Input: part model. Units: mm. Frame: model coordinates. A direction names the side the tool comes from. Coordinates: 2 decimals unless noted, no trailing zeros. Write each loop counter-clockwise with the first axis right and the second up, starting at its lowest first coordinate (ties: lowest second). Pieces come first, ordered by that corner, then holes. Notation, with made-up numbers: (6, 0) - (51, 0) arc R23 cw to (51, 19) - close; hole circle Ø9 at (78.5, 29). An arc over 180 degrees is marked (long way). Use CSV: the item, a comma, the result in double quotes.
Autodesk Fusion 360 part; units mm, degrees
sketch "Sketch1" plane through (0, 0, 0) normal (0, 0, 1) x (1, 0, 0)
  line L0 (-50.8, 50.8) -> (50.8, 50.8)
  line L1 (50.8, 50.8) -> (50.8, -50.8)
  line L2 (50.8, -50.8) -> (-50.8, -50.8)
  line L3 (-50.8, -50.8) -> (-50.8, 50.8)
  line L4 (-50.8, 50.8) -> (50.8, -50.8) construction
  line L5 (50.8, 50.8) -> (-50.8, -50.8) construction
  circle A0 centre (0, 0) radius 27.43
  line L6 (0, 0) -> (-40.48, 0) construction
  line L7 (-40.48, 0) -> (-40.48, -40.48) construction
  line L8 (-40.48, -40.48) -> (0, -40.48) construction
  line L9 (0, -40.48) -> (0, 0) construction
  circle A1 centre (-40.48, -40.48) radius 1.985
  circle A2 centre (-40.48, 40.48) radius 1.985
  circle A3 centre (40.48, 40.48) radius 1.985
  circle A4 centre (40.48, -40.48) radius 1.985
  circle A5 centre (0, 0) radius 45
  dimension "d1" = 101.6
  dimension "d2" = 101.6
  dimension "d3" = 54.86
  dimension "d4" = 40.48
  dimension "d5" = 40.48
  dimension "d6" = 3.97
extrude "Extrude1" add sketch "Sketch1" against normal blind 0.74 contours L0 L1 L2 L3 | A5
extrude "Extrude2" add sketch "Sketch1" along normal blind 6.65 contours A5
sketch "Sketch2" plane through (0, 0, 6.65) normal (0, 0, 1) x (-1, 0, 0)
  circle A0 centre (0, 0) radius 27.43
  circle A1 centre (0, 0) radius 45
  circle A2 centre (0, 0) radius 45
  circle A3 centre (-40.48, 40.48) radius 1.985
  circle A4 centre (40.48, 40.48) radius 1.985
  circle A5 centre (40.48, -40.48) radius 1.985
  circle A6 centre (-40.48, -40.48) radius 1.985
  line L0 (50.8, 50.8) -> (-50.8, 50.8)
  line L1 (-50.8, 50.8) -> (-50.8, -50.8)
  line L2 (-50.8, -50.8) -> (50.8, -50.8)
  line L3 (50.8, -50.8) -> (50.8, 50.8)
extrude "Extrude3" add sketch "Sketch2" along normal blind 0.74 contours A1 A2 | L0 L1 L2 L3
(1) Ray query, probe 1 along Y at (x, z) = (-40.48, 6.9) (3 decimals); probe 2 along Y at (x, z) = (0, 3.25). Return the intervals inside material, ascending. Write a range as from..to.
Check values:
probe 1,"-50.8..-42.465, -38.495..38.495, 42.465..50.8"
probe 2,"-45..-27.43, 27.43..45"
(2) Cut plane C-C on y = -10.5. Return loops of the section in (x, z), and give its area (3 significant figures).
Check values:
outline,"(-50.8, -0.74) - (-25.34, -0.74) - (-25.34, 7.39) - (-50.8, 7.39) - (-50.8, 6.65) - (-43.76, 6.65) - (-43.76, 0) - (-50.8, 0) - close; (25.34, -0.74) - (50.8, -0.74) - (50.8, 0) - (43.76, 0) - (43.76, 6.65) - (50.8, 6.65) - (50.8, 7.39) - (25.34, 7.39) - close"
area,"320 mm^2"
(3) Pin query (flat end, axial travel): pin 1 Ø5 at (x, y) = (-40.48, -40.48) entering from -Z; pin 2 Ø1 at (y, z) = (34, 2) entering from +X; pin 3 Ø3 at (x, z) = (19.5, 3) entering from -Y; pin 4 Ø1 at (y, z) = (33.5, 6) entering from -X. Return the tip coordinate at first contact, or that it passes through.
Check values:
pin 1,"z = -0.74"
pin 2,"x = 30.05"
pin 3,"y = -41.24"
pin 4,"x = -30.59"
(4) Draft query along Y for faces 1 (the flat face through (-22, 22, 7.39)), 2 (the cylindrical face through (20.765, 39.923, 3.278)), 3 (the cylindrical face through (40.738, 42.448, 7.015)). Return one class per face: pulls with the +Y half, pulls with the -Y half, needs draft (parallel to the pull), parting line crosses it, or undercut.
Check values:
face 1,"needs draft"
face 2,"parting line crosses it"
face 3,"undercut"
(5) Reachability of faces 4 (the flat face through (1, -46, 6.65)), 5 (the cylindrical face through (41.943, -39.138, 7.015)) from +Z, -Z, +X, -X, +Y, -Y: full face, straight path, thin tool, end or side. Return the list, or none.
Check values:
face 4,"none"
face 5,"+Z, -Z"
(6) Cut plane D-D on z = 3.75. Return loops of the section in (x, y), and give its area (3 significant figures).
Check values:
outline,"circle Ø90 at (0, 0); hole circle Ø54.86 at (0, 0)"
area,"4,000 mm^2"
(7) Cut plane A-A on y = 40.48. Return loops of the section in (x, z) (3 decimals).
Check values:
outline,"(-50.8, -0.74) - (-42.465, -0.74) - (-42.465, 0) - (-50.8, 0) - close; (-50.8, 6.65) - (-42.465, 6.65) - (-42.465, 7.39) - (-50.8, 7.39) - close; (-38.495, -0.74) - (38.495, -0.74) - (38.495, 0) - (19.656, 0) - (19.656, 6.65) - (38.495, 6.65) - (38.495, 7.39) - (-38.495, 7.39) - (-38.495, 6.65) - (-19.656, 6.65) - (-19.656, 0) - (-38.495, 0) - close; (42.465, -0.74) - (50.8, -0.74) - (50.8, 0) - (42.465, 0) - close; (42.465, 6.65) - (50.8, 6.65) - (50.8, 7.39) - (42.465, 7.39) - close"
